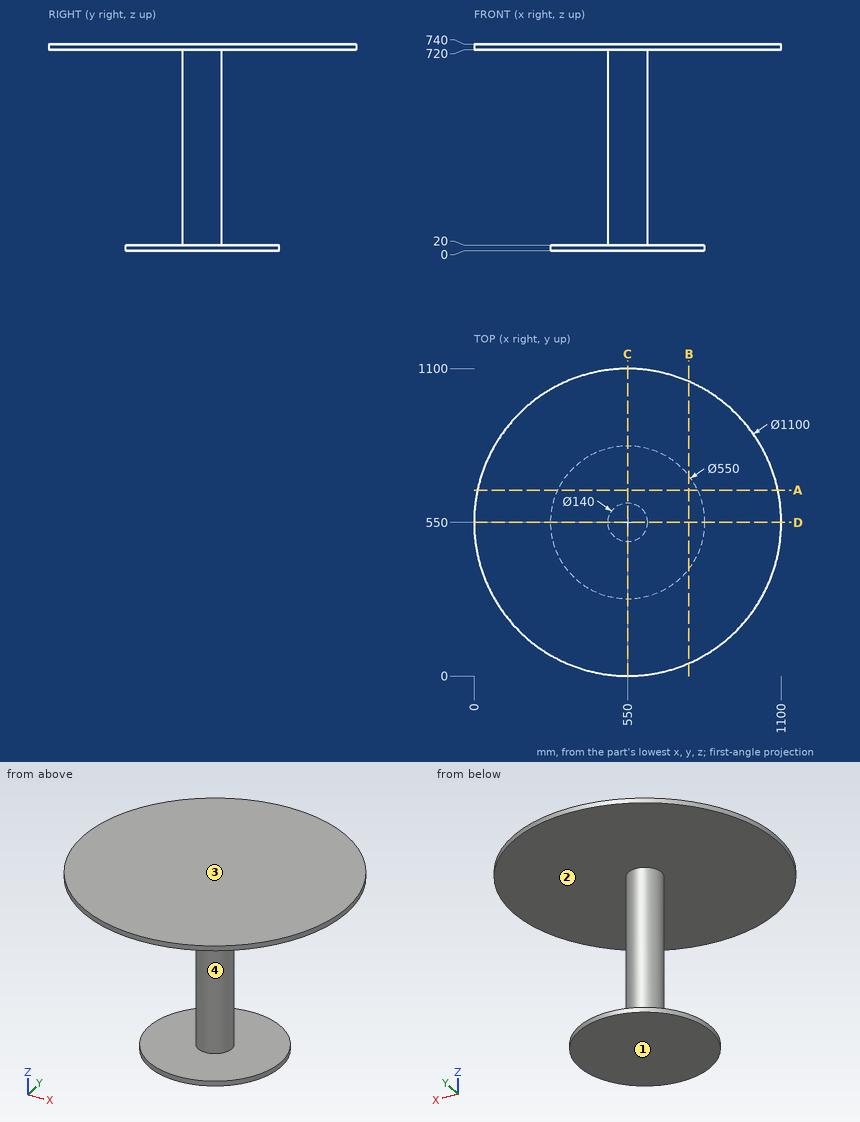
Input: dimensioned drawing with shaded views. Units: mm. Origin: part minimum x, y, z. Coordinates: 2 decimals unless noted, no trailing zeros. Loops run counter-clockwise (first coordinate to the right, second up) from the corner with the lowest first, then second, coordinate; pieces in that order, holes last. Notation, with made-up numbers: M 25,49 L 61,49 A13 ccw 61,63 Z; hole C 9.5,-33 d10. An arc over 180 degrees is marked long. Use a Markdown table: item, result. Add a question column.
Q1. Material intervals for L1, parallel to Z at x = 437, y = 752; L2, parallel to Z at x = 712, y = 93; L3, parallel to Y at x = 525.5, z = 553.5, sorted ascending.
Q2. Section query B-B, the plane x = 769. Return loops of the section in (y, z), and give its area (3 significant figures).
Q3. Section query C-C, the plane x = 550. Return loops of the section in (y, z).
Q4. First-contact query: pin 1 (5 mm diameter, centred on x = 514, z = 465.5, fed in from +Y). Flat tip, straight axial feed; report the tip coordinate or a pass-through.
Q5. Draft query along Z for the marked faces 1, 2, 3 and 4. Return one class per face: pulls with the +Z half, pulls with the -Z half, needs draft (parallel to the pull), parting line crosses it, or undercut.
Q6. Section query A-A, the plane y = 665.5. Return loops of the section in (x, z), and give its area (3 significant figures).
Result:
| question | item | result |
|---|---|---|
| 1 | L1 | z = 0 to 20, 720 to 740 |
| 1 | L2 | z = 720 to 740 |
| 1 | L3 | y = 484.43 to 615.57 |
| 2 | outline | M 45.48,720 L 1054.52,720 L 1054.52,740 L 45.48,740 Z; M 383.68,0 L 716.32,0 L 716.32,20 L 383.68,20 Z |
| 2 | area | 26,800 mm2 |
| 3 | outline | M 0,720 L 480,720 L 480,20 L 275,20 L 275,0 L 825,0 L 825,20 L 620,20 L 620,720 L 1100,720 L 1100,740 L 0,740 Z |
| 4 | pin 1 | stops at y = 611.46 |
| 5 | face 1 | pulls with the -Z half |
| 5 | face 2 | undercut |
| 5 | face 3 | pulls with the +Z half |
| 5 | face 4 | undercut |
| 6 | outline | M 12.26,720 L 1087.74,720 L 1087.74,740 L 12.26,740 Z; M 300.43,0 L 799.57,0 L 799.57,20 L 300.43,20 Z |
| 6 | area | 31,500 mm2 |
